Source: CAD feature listing. Evaluate the final solid. Frame: model axes, mm. A direction names the side the tool comes from. Give positions to 0.01 mm unless a question says otherwise; leave off trailing zeros. Loops run counter-clockwise (first coordinate to the right, second up) from the corner with the lowest first, then second, coordinate; pieces in that order, holes last.
```python
from build123d import *

# Parameters (mm, degrees)
EXTRUDE_1_DEPTH          = 100
EXTRUDE_1_DEPTH_BACK     = 100
SKETCH_1_R               = 83
SHELL_1_T                = -1
SKETCH_2_R               = 82.5
SKETCH_2_R_2             = 65
EXTRUDE_2_DEPTH          = 2
CUT_EXTRUDE_1_DEPTH      = 28
SKETCH_5_W               = 70
SKETCH_5_H               = 60
CUT_EXTRUDE_2_DEPTH      = 155.201167311
PATTERN_CIRCULAR_1_COUNT = 4
SKETCH_6_W               = 40
SKETCH_6_H               = 5
CUT_EXTRUDE_3_DEPTH      = 30
CUT_EXTRUDE_4_REACH      = 210.235
SKETCH_7_R               = 1.6


with BuildPart() as part:
    # 草图1 → 凸台-拉伸1 (new, two sides: drawn at the far end of the back side and taken through both)
    with BuildSketch(Plane.XY.offset(-EXTRUDE_1_DEPTH_BACK)):
        Circle(SKETCH_1_R)
    extrude(amount=EXTRUDE_1_DEPTH + EXTRUDE_1_DEPTH_BACK)

    # 抽壳1
    shell_1_openings = [part.faces().sort_by_distance(p)[0] for p in [
        (0, 0, -100),
        (0, 0, 100),
    ]]
    offset(amount=SHELL_1_T, openings=shell_1_openings, kind=Kind.INTERSECTION)

    # 草图2 → 凸台-拉伸2 (add)
    with BuildSketch(Plane.XY.offset(70)):
        Circle(SKETCH_2_R)
        Circle(SKETCH_2_R_2, mode=Mode.SUBTRACT)
    extrude(amount=EXTRUDE_2_DEPTH)

    # 草图3 → 切除-拉伸1 (cut)
    with BuildSketch(Plane.XY.offset(100)):
        with BuildLine():
            Line((43.273355415, 70.826666667), (-43.273355415, 70.826666667))
            ThreePointArc((-43.273355415, 70.826666667), (0, 83), (43.273355415, 70.826666667))
        make_face()
    extrude(amount=-CUT_EXTRUDE_1_DEPTH, mode=Mode.SUBTRACT)

    # 草图5 → 切除-拉伸2 (cut, symmetric)
    with BuildSketch(Plane(origin=(0, 0, 0), x_dir=(1, 0, 0), z_dir=(0, 1, 0))):
        with Locations((0, 70)):
            Rectangle(SKETCH_5_W, SKETCH_5_H)
    cut_extrude_2 = extrude(amount=CUT_EXTRUDE_2_DEPTH, both=True, mode=Mode.SUBTRACT)

    # 阵列(圆周)1: 切除-拉伸2 ×4 about axis
    pattern_circular_1_axis = Axis((0, 0, -100), (0, 0, 1))
    for i in range(1, PATTERN_CIRCULAR_1_COUNT):
        add(cut_extrude_2.rotate(pattern_circular_1_axis, i * 360 / PATTERN_CIRCULAR_1_COUNT), mode=Mode.SUBTRACT)

    # 草图6 → 切除-拉伸3 (cut)
    with BuildSketch(Plane(origin=(0, 0, 72), x_dir=(1, 0, 0), z_dir=(0, 0, -1))):
        Polygon((-64.045172024, 60.070508076), (-84.045172024, 25.429491924), (-79.715045005, 22.929491924), (-59.715045005, 57.570508076), align=None)
        with Locations((0, -83)):
            Rectangle(SKETCH_6_W, SKETCH_6_H)
        Polygon((84.045172024, 25.429491924), (64.045172024, 60.070508076), (59.715045005, 57.570508076), (79.715045005, 22.929491924), align=None)
    extrude(amount=CUT_EXTRUDE_3_DEPTH, mode=Mode.SUBTRACT)

    # 草图7 → 切除-拉伸4 (cut, up to next)
    with BuildSketch(Plane.XY.offset(72), mode=Mode.PRIVATE) as cut_extrude_4_sk1:
        with Locations((0, 68.5)):
            Circle(SKETCH_7_R)
    cut_extrude_4_tool1 = extrude(cut_extrude_4_sk1.sketch, amount=-CUT_EXTRUDE_4_REACH, mode=Mode.PRIVATE) & part.part
    # 草图7 → 切除-拉伸4 (cut, up to next)
    with BuildSketch(Plane.XY.offset(72), mode=Mode.PRIVATE) as cut_extrude_4_sk2:
        with Locations((-68.5, 0)):
            Circle(SKETCH_7_R)
    cut_extrude_4_tool2 = extrude(cut_extrude_4_sk2.sketch, amount=-CUT_EXTRUDE_4_REACH, mode=Mode.PRIVATE) & part.part
    # 草图7 → 切除-拉伸4 (cut, up to next)
    with BuildSketch(Plane.XY.offset(72), mode=Mode.PRIVATE) as cut_extrude_4_sk3:
        with Locations((0, -68.5)):
            Circle(SKETCH_7_R)
    cut_extrude_4_tool3 = extrude(cut_extrude_4_sk3.sketch, amount=-CUT_EXTRUDE_4_REACH, mode=Mode.PRIVATE) & part.part
    # 草图7 → 切除-拉伸4 (cut, up to next)
    with BuildSketch(Plane.XY.offset(72), mode=Mode.PRIVATE) as cut_extrude_4_sk4:
        with Locations((68.5, 0)):
            Circle(SKETCH_7_R)
    cut_extrude_4_tool4 = extrude(cut_extrude_4_sk4.sketch, amount=-CUT_EXTRUDE_4_REACH, mode=Mode.PRIVATE) & part.part
    add(cut_extrude_4_tool1.solids().sort_by_distance((0, 68.5, 72))[0], mode=Mode.SUBTRACT)
    add(cut_extrude_4_tool2.solids().sort_by_distance((-68.5, 0, 72))[0], mode=Mode.SUBTRACT)
    add(cut_extrude_4_tool3.solids().sort_by_distance((0, -68.5, 72))[0], mode=Mode.SUBTRACT)
    add(cut_extrude_4_tool4.solids().sort_by_distance((68.5, 0, 72))[0], mode=Mode.SUBTRACT)


solid = part.part
```
(1) Section A-A, the plane z = -80.5. Return the cut outline in (x, y).
A:
outline: (-75.26, -35) arc R83 ccw to (-35, -75.26) - (-35, -74.16) arc R82 cw to (-74.16, -35) - close; (-75.26, 35) - (-74.16, 35) arc R82 cw to (-35, 74.16) - (-35, 75.26) arc R83 ccw to start; (35, -75.26) arc R83 ccw to (75.26, -35) - (74.16, -35) arc R82 cw to (35, -74.16) - close; (35, 74.16) arc R82 cw to (74.16, 35) - (75.26, 35) arc R83 ccw to (35, 75.26) - close
(2) Reachability of faces 1 (the flat face through (-37, -55, 70)), 2 (the flat face through (-71, -42, 72)), 3 (the flat face through (57, -60, -100)), 4 (the flat face through (71, -42, 42)) from +Z, -Z, +X, -X, +Y, -Y: full face, straight path, thin tool, end or side. Return the list, or none.
A:
face 1: -Z
face 2: -X, -Y
face 3: -Z, +X, -X, +Y, -Y
face 4: +X, -Y
(3) First-contact query: pin 1 (10 mm diameter, centred on y = 41, z = -45, fed in from +X); pin 2 (0.6 mm diameter, centred on x = -42, z = 82.5, fed in from +Y); pin 3 (8 mm diameter, centred on x = 36.5, z = 2, fed in from -Y). Flat tips, straight axial feed; report the tip coordinate or a pass-through.
A:
pin 1: stops at x = 74.79
pin 2: stops at y = 70.83
pin 3: stops at y = -76.37
(4) Section D-D, the plane z = 2. Return the cut outline in (x, y), then the cut area to 3 significant figures.
A:
outline: circle Ø166 at (0, 0); hole circle Ø164 at (0, 0)
area: 518 mm2
(5) Section C-C, the plane y = -14.5. Return the cut outline in (x, z).
A:
outline: (-81.72, -40) - (-80.71, -40) - (-80.71, 70) - (-63.36, 70) - (-63.36, 72) - (-80.71, 72) - (-80.71, 100) - (-81.72, 100) - close; (63.36, 70) - (80.71, 70) - (80.71, -40) - (81.72, -40) - (81.72, 100) - (80.71, 100) - (80.71, 72) - (63.36, 72) - close
(6) Mould query, pull axis Y, two halves, no side actions, for faces 5 (the flat face through (24, -61, 72)), 6 (the flat face through (-58.2, -58, -100)), 7 (the flat face through (67.446, -44.18, 70.403)). Classes: pulls with the +Y half, pulls with the -Y half, needs draft (parallel to the pull), parting line crosses it, or undercut.
A:
face 5: undercut
face 6: needs draft
face 7: pulls with the -Y half
(7) Ray query, line 1 along X through (y, z) = (0, 86); line 2 along Y through (x, z) = (-31.5, 24); line 3 along X through (y, z) = (-68.5, 71.35). Return the intervals inside material, ascending.
A:
line 1: x = -83 to -82, 82 to 83
line 2: y = -76.79 to -75.71, 75.71 to 76.79
line 3: x = -46.87 to -1.6, 1.6 to 46.87
(8) Section B-B, the plane x = -56. Return the cut outline in (y, z), then the cut area to 3 significant figures.
A:
outline: (-61.26, -100) - (-59.9, -100) - (-59.9, 70) - (-33, 70) - (-33, 72) - (-59.9, 72) - (-59.9, 100) - (-61.26, 100) - close; (33, 70) - (59.9, 70) - (59.9, -100) - (61.26, -100) - (61.26, 100) - (59.9, 100) - (59.9, 72) - (33, 72) - close
area: 652 mm2
